Geometry: see drawing. Coordinates: mm, zero at the bounding-box minimum. A direction names the side the tool comes from. Round coordinates to 2 decimals unless told otherwise and drop trailing zeros. Loops run counter-clockwise (first coordinate to the right, second up) from the corner with the lowest first, then second, coordinate; pieces in that order, holes last. Notation, with made-up numbers: (-40, 71) - (-3, 71) arc R30 cw to (-3, 103) - close; hole circle Ø8 at (19.5, 35.5). An arc over 180 degrees is marked (long way). Use CSV: the item, a comma, the result in double quotes. Start each with the question number.
1. Cut plane B-B (y = 3.25). Return loops of the section in (x, z), and give its area (3 significant figures).
2. Access query for the marked faces 1, 2 and 3. Directions: +Z, -Z, +X, -X, +Y, -Y. A direction counts if a zero-diameter tool reaches every point of the face in a straight line with its end or side. Return the directions, or none.
3. Material intervals for probe 1 along Y at (x, z) = (60, 30.85); probe 2 along X at (y, z) = (7.75, 31); probe 3 along X at (y, z) = (12.25, 17.5), sorted ascending. Write a range as from..to.
4. Cut plane C-C (y = 8). Return loops of the section in (x, z).
5. Cut plane A-A (x = 60). Return loops of the section in (y, z).
6. Pin query (flat end, axial travel): P1, Ø4.5, axis at x = 56, y = 9, coming from the -Z side; P2, Ø4.5, axis at x = 60, y = 8, coming from the -Z side; P3, Ø1, axis at y = 1.5, z = 20, coming from the -X side. Return the tip coordinate at first contact, or that it passes through.
7. Pull-direction query (Y, two-part tool) for the marked faces 4, 5 and 6; classes: +Y half, -Y half, draft (parallel to the pull), parting line (faces both ways), or undercut.
8. Cut plane D-D (z = 32.5). Return loops of the section in (x, y).
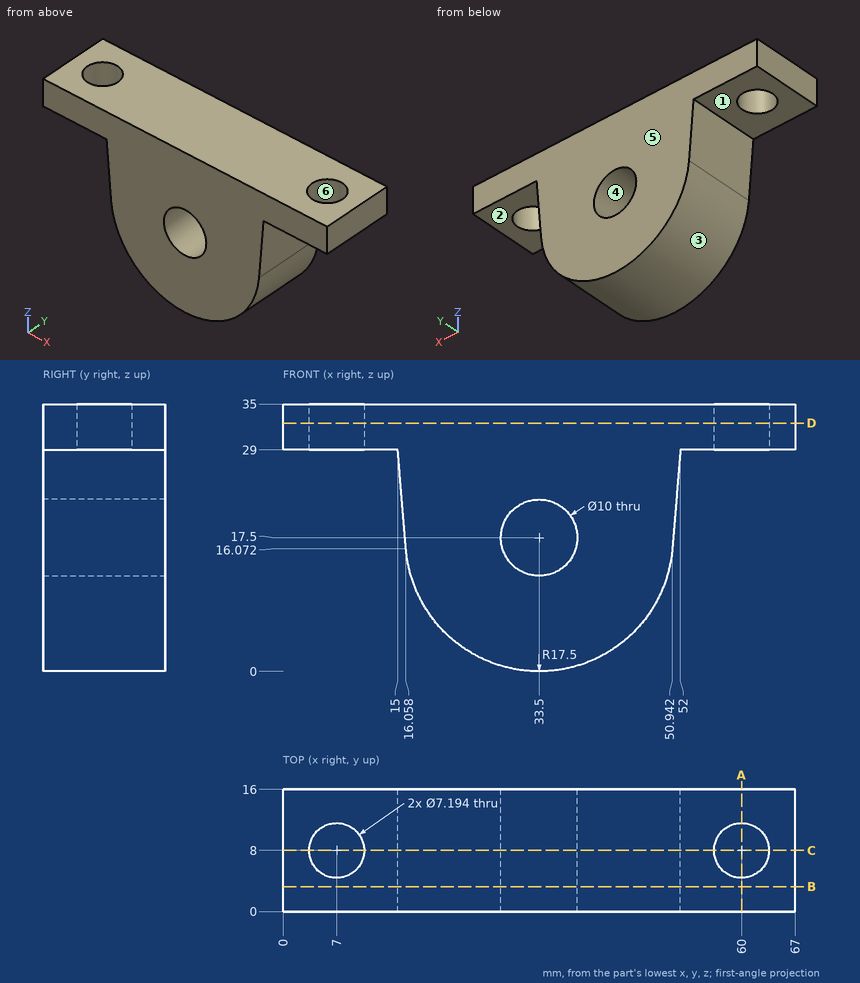
Established:
1,outline,"(0, 29) - (15, 29) - (16.06, 16.07) arc R17.5 ccw to (50.94, 16.07) - (52, 29) - (67, 29) - (67, 35) - (0, 35) - close; hole circle Ø10 at (33.5, 17.5)"
1,area,"1,220 mm2"
2,face 1,"-Z, -X, +Y, -Y"
2,face 2,"-Z, +X, +Y, -Y"
2,face 3,"-Z, +Y, -Y"
3,probe 1,"y = 0..4.4, 11.6..16"
3,probe 2,"x = 0..3.41, 10.59..56.41, 63.59..67"
3,probe 3,"x = 15.94..28.5, 38.5..51.06"
4,outline,"(0, 29) - (3.4, 29) - (3.4, 35) - (0, 35) - close; (10.6, 29) - (15, 29) - (16.06, 16.07) arc R17.5 ccw to (50.94, 16.07) - (52, 29) - (56.4, 29) - (56.4, 35) - (10.6, 35) - close; (63.6, 29) - (67, 29) - (67, 35) - (63.6, 35) - close; hole circle Ø10 at (33.5, 17.5)"
5,outline,"(0, 29) - (4.4, 29) - (4.4, 35) - (0, 35) - close; (11.6, 29) - (16, 29) - (16, 35) - (11.6, 35) - close"
6,P1,"stops at z = 29"
6,P2,"passes through"
6,P3,"stops at x = 15.7"
7,face 4,"draft"
7,face 5,"+Y half"
7,face 6,"undercut"
8,outline,"(0, 0) - (67, 0) - (67, 16) - (0, 16) - close; hole circle Ø7.19 at (7, 8); hole circle Ø7.19 at (60, 8)"
